```python
from build123d import *

# Parameters (mm, degrees)
F0_W     = 63.20139
F0_H     = 47.793298
F0_R     = 5.383544
F0_R_2   = 6.809705
F0_R_3   = 5.839267
F0_R_4   = 7.460797
F1_DEPTH = 2
F3_DEPTH = 50


with BuildPart() as f1:
    # F0 (on Top) → F1 (new body)
    with BuildSketch(Plane.XY):
        Rectangle(F0_W, F0_H)
        with Locations((-25.030309, -17.485425)):
            Circle(F0_R, mode=Mode.SUBTRACT)
        with Locations((19.828575, -15.185272)):
            Circle(F0_R_2, mode=Mode.SUBTRACT)
        with Locations((-24.514884, 13.153892)):
            Circle(F0_R_3, mode=Mode.SUBTRACT)
        with Locations((21.219891, 13.936961)):
            Circle(F0_R_4, mode=Mode.SUBTRACT)
    extrude(amount=F1_DEPTH)

    # F2 (on face) → F3 (join)
    with BuildSketch(Plane.XZ.offset(23.896649)):
        Polygon((12.217186, 2), (12.217186, 9.05502), (-16.335363, 19.447298), (-16.335363, 2), align=None)
    extrude(amount=-F3_DEPTH)


solid = f1.part
```
Here's how the part is built. I have some questions about the finished solid (model axes, mm). A direction names the side the tool comes from. Round coordinates to 2 decimals unless told otherwise and drop trailing zeros. Write each loop counter-clockwise with the first axis right and the second up, starting at its lowest first coordinate (ties: lowest second). Pieces come first, ordered by that corner, then holes.
Q1. If we section it at D-D on x = 16: Write out the boundary of the cut face in (y, z).
Q2. Please list where these lines run through material, in increasing order: probe 1 along X at (y, z) = (11, 4.25); probe 2 along Z at (x, y) = (3.5, -14.5); probe 3 along Z at (x, y) = (13.5, 10.5).
Q3. If we section it at C-C on y = -7: Write out the boundary of the cut face in (x, z).
Q4. Which directions (+Z, -Z, +X, -X, +Y, -Y) give clear straight access to the entire face, cutting with the end or side of a thin tool? Please do faces 4 (the flat face through (-2, 25, 2)), 5 (the flat face through (-31.601, 0, 1)), 6 (the flat face through (-16.335, 1, 11)), 7 (the flat face through (12.217, 1, 5)).
Q5. If we section it at B-B on y = 16: Write out the boundary of the cut face in (x, z), plus the area to 3 significant figures.
Q6. If we mould it in two halves opening along X, with no side actions, what happens to faces 1 (the flat face through (-7, -23.897, 8)), 2 (the cylindrical face through (-21.82, 7.973, 0.986)), 3 (the flat face through (31.601, 0, 1))? For each: +X half, -X half, draft (parallel to the pull), parting line (faces both ways), or undercut.
Q7. Will these pins go through, and if not, where does the flat tip stop? P1, Ø12, axis at x = -27, y = -1, coming from the +Z side; P2, Ø5, axis at y = 2.5, z = 5, coming from the +X side; P3, Ø0.7, axis at x = -8, y = 24.5, coming from the -Z side.
Q8. If we section it at A-A on x = -25: Write out the boundary of the cut face in (y, z).
Answer below:
1. outline: (-23.9, 0) - (-20.82, 0) - (-20.82, 2) - (-23.9, 2) - close; (-9.55, 0) - (8.61, 0) - (8.61, 2) - (-9.55, 2) - close; (19.27, 0) - (23.9, 0) - (23.9, 2) - (19.27, 2) - close
2. probe 1: x = -16.34 to 12.22
2. probe 2: z = 0 to 12.23
2. probe 3: z = 0 to 2
3. outline: (-31.6, 0) - (31.6, 0) - (31.6, 2) - (12.22, 2) - (12.22, 9.06) - (-16.34, 19.45) - (-16.34, 2) - (-31.6, 2) - close
4. face 4: -Z, +X, -X, +Y
4. face 5: +Z, -Z, -X, +Y, -Y
4. face 6: +Z, -X, +Y, -Y
4. face 7: +Z, +X, +Y, -Y
5. outline: (-31.6, 0) - (-29.61, 0) - (-29.61, 2) - (-31.6, 2) - close; (-19.42, 0) - (14.05, 0) - (14.05, 2) - (12.22, 2) - (12.22, 9.06) - (-16.34, 19.45) - (-16.34, 2) - (-19.42, 2) - close; (28.39, 0) - (31.6, 0) - (31.6, 2) - (28.39, 2) - close
5. area: 427 mm2
6. face 1: draft
6. face 2: undercut
6. face 3: +X half
7. P1: stops at z = 2
7. P2: stops at x = 12.22
7. P3: stops at z = 2
8. outline: (-23.9, 0) - (-22.87, 0) - (-22.87, 2) - (-23.9, 2) - close; (-12.1, 0) - (7.33, 0) - (7.33, 2) - (-12.1, 2) - close; (18.97, 0) - (23.9, 0) - (23.9, 2) - (18.97, 2) - close
